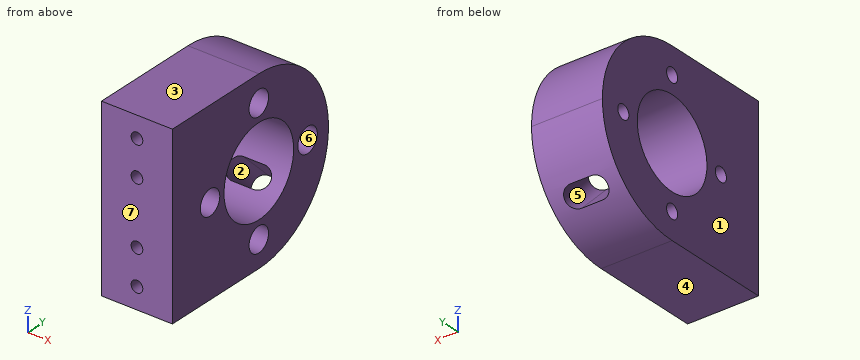
from build123d import *

# Parameters (mm, degrees)
SKIZZE1_W                       = 20
SKIZZE1_H                       = 50
AUFSATZ_LINEAR_AUSTRAGEN1_DEPTH = 56
SKIZZE2_R                       = 12.5
SKIZZE2_R_2                     = 2
SCHNITT_LINEAR_AUSTRAGEN1_DEPTH = 65.505813691
SKIZZE3_R                       = 1.65
SCHNITT_LINEAR_AUSTRAGEN2_DEPTH = 15
SKIZZE6_R                       = 3.5
SCHNITT_LINEAR_AUSTRAGEN5_DEPTH = 10
CUT_EXTRUDE1_DEPTH              = 17


with BuildPart() as part:
    # Skizze1 → Aufsatz-Linear austragen1 (new body)
    with BuildSketch(Plane(origin=(0, 0, 0), x_dir=(1, 0, 0), z_dir=(0, 1, 0))):
        Rectangle(SKIZZE1_W, SKIZZE1_H)
    extrude(amount=AUFSATZ_LINEAR_AUSTRAGEN1_DEPTH)

    # Skizze2 → Schnitt-Linear austragen1 (cut, through all)
    with BuildSketch(Plane.ZY.offset(10)):
        with BuildLine():
            Line((-25, 56), (-25, 31))
            ThreePointArc((-25, 31), (-17.677669509, 48.67766955), (5.8e-08, 56))
            Line((5.8e-08, 56), (-25, 56))
        make_face()
        with BuildLine():
            ThreePointArc((5.8e-08, 56), (17.67766955, 48.677669509), (25, 31))
            Line((25, 31), (25, 56))
            Line((25, 56), (5.8e-08, 56))
        make_face()
        with Locations((0, 31)):
            Circle(SKIZZE2_R)
        with Locations((17.5, 31)):
            Circle(SKIZZE2_R_2)
        with Locations((0, 48.5)):
            Circle(SKIZZE2_R_2)
        with Locations((0, 13.5)):
            Circle(SKIZZE2_R_2)
        with Locations((-17.5, 31)):
            Circle(SKIZZE2_R_2)
    extrude(amount=-SCHNITT_LINEAR_AUSTRAGEN1_DEPTH, mode=Mode.SUBTRACT)

    # Skizze3 → Schnitt-Linear austragen2 (cut)
    with BuildSketch(Plane.XZ):
        with Locations(Location((0, 19, 0), (0, 0, 270))):
            Circle(SKIZZE3_R)
        with Locations(Location((0, 9, 0), (0, 0, 270))):
            Circle(SKIZZE3_R)
        with Locations(Location((0, -9, 0), (0, 0, 90))):
            Circle(SKIZZE3_R)
        with Locations(Location((0, -19, 0), (0, 0, 90))):
            Circle(SKIZZE3_R)
    extrude(amount=-SCHNITT_LINEAR_AUSTRAGEN2_DEPTH, mode=Mode.SUBTRACT)

    # Skizze6 → Schnitt-Linear austragen5 (cut)
    with BuildSketch(Plane(origin=(10, 0, 0), x_dir=(0, 0, -1), z_dir=(1, 0, 0))):
        with Locations((17.5, 31)):
            Circle(SKIZZE6_R)
        with Locations((0.001666066, 13.498333934)):
            Circle(SKIZZE6_R)
        with Locations((-17.5, 30.996667867)):
            Circle(SKIZZE6_R)
        with Locations((-0.001666066, 48.498333934)):
            Circle(SKIZZE6_R)
    extrude(amount=-SCHNITT_LINEAR_AUSTRAGEN5_DEPTH, mode=Mode.SUBTRACT)

    # Sketch1 → Cut-Extrude1 (cut)
    with BuildSketch(Plane(origin=(0, 33.17766953, -33.17766953), x_dir=(-1, 0, 0), z_dir=(0, 0.7071067811865537, -0.7071067811865414))):
        with BuildLine():
            Line((-3, 25.5), (3, 25.5))
            ThreePointArc((3, 25.5), (6, 22.5), (3, 19.5))
            Line((3, 19.5), (-3, 19.5))
            ThreePointArc((-3, 19.5), (-6, 22.5), (-3, 25.5))
        make_face()
    extrude(amount=-CUT_EXTRUDE1_DEPTH, mode=Mode.SUBTRACT)


solid = part.part
CAD build for the part. Positions are in the model's coordinates, mm. Face numbers are marked on the shaded views. A direction names the side the tool comes from. Round coordinates to 2 decimals unless told otherwise and drop trailing zeros. Order: outer loops, then holes, each group sorted by start corner. A loop starts at its lowest first (then second) coordinate and runs counter-clockwise, first axis right, second up. Notation, with made-up numbers: (13, -25.75) -> (32, -25.75) arc R17 ccw to (32, -11.75) -> close; hole circle Ø9 at (1, 7). An arc over 180 degrees is marked (long way). Write item = value, one per line. Start each with the question number.
(1) Which spindle directions (+Z, -Z, +X, -X, +Y, -Y) get a long thin tool onto all of the face, cutting with end or side? Do the marked faces 5, 6 and 7. Say none if no direction does.
(2) Cut at C-C, the plane y = 23. List the corners of the cut face in (x, z), then the cut area to 3 significant figures.
(3) Pin check, flat tips, straight feed: P1, Ø4, axis at x = 0, z = -19, coming from the -Y side; P2, Ø10, axis at y = 33.5, z = -5.5, coming from the -X side; P3, Ø2.5, axis at x = 0, z = 9, coming from the -Y side; P4, Ø2, axis at x = -4.5, z = -17.5, coming from the +Y side. Stop position of each tip, or through.
(4) Cut at B-B, the plane z = -5. List the corners of the cut face in (x, y), then the cut area to 3 significant figures.
(5) Cut at D-D, the plane x = 8.5. List the corners of the cut face in (y, z).
(6) Probe line 1 (Y direction, x = -3, z = -11); line 2 (Y direction, x = -4, z = 9); line 3 (Y direction, x = 8.75, z = -8). List the from-to ranges inside material, lowest first. Write a range as [from, to].
(7) Pull direction Z, two halves, no side cores. Call the marked faces 1, 2, 3 and 4: released by +Z, released by -Z, zero draft, split by the parting line, or undercut.
(8) Cut at A-A, the plane y = 4.5. List the corners of the cut face in (x, z).
Model answer:
q1.face_5 = none
q1.face_6 = +X
q1.face_7 = +Z, -Z, +X, -X, -Y
q2.outline = (-10, -25) -> (10, -25) -> (10, -9.6) -> (-10, -9.6) -> close; (-10, 9.6) -> (10, 9.6) -> (10, 25) -> (-10, 25) -> close
q2.area = 616 mm2
q3.P1 = 0
q3.P2 = through
q3.P3 = 15
q3.P4 = 47.21
q4.outline = (-10, 0) -> (10, 0) -> (10, 19.54) -> (-10, 19.54) -> close; (-10, 42.46) -> (10, 42.46) -> (10, 55.49) -> (-10, 55.49) -> close
q4.area = 652 mm2
q5.outline = (0, -25) -> (31, -25) arc R25 ccw to (31, 25) -> (0, 25) -> close; hole circle Ø7 at (13.5, 0); hole circle Ø25 at (31, 0); hole circle Ø7 at (31, -17.5); hole circle Ø7 at (31, 17.5); hole circle Ø7 at (48.5, 0)
q6.line_1 = [0, 25.06], [36.94, 38.58], [47.06, 53.45]
q6.line_2 = [0, 22.33], [39.67, 54.32]
q6.line_3 = [0, 21.4], [40.6, 54.69]
q7.face_1 = zero draft
q7.face_2 = undercut
q7.face_3 = released by +Z
q7.face_4 = released by -Z
q8.outline = (-10, -25) -> (10, -25) -> (10, 25) -> (-10, 25) -> close; hole circle Ø3.3 at (0, -19); hole circle Ø3.3 at (0, -9); hole circle Ø3.3 at (0, 9); hole circle Ø3.3 at (0, 19)
